Model file for the job. Use its own axes, mm. Face numbers are marked on the shaded views. A direction names the side the tool comes from. Give positions to 0.01 mm unless a question says otherwise; leave off trailing zeros. Loops run counter-clockwise (first coordinate to the right, second up) from the corner with the lowest first, then second, coordinate; pieces in that order, holes last. Notation, with made-up numbers: (-6.75, 56) - (1.25, 56) arc R28 ccw to (1.25, 75) - close; hole circle Ø1 at (58, 83.25). An arc over 180 degrees is marked (long way). Use a Markdown table: item, result.
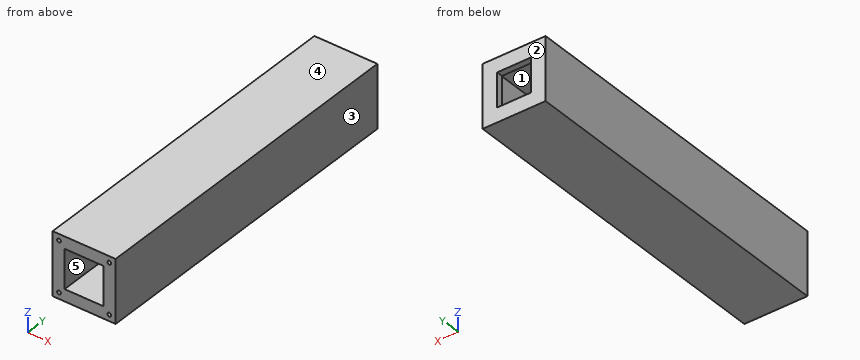
from build123d import *

# Parameters (mm, degrees)
SKETCH_1_W          = 10
SKETCH_1_H          = 10
SKETCH_1_W_2        = 6.2
SKETCH_1_H_2        = 6.2
EXTRUDE_1_DEPTH     = 54
EXTRUDE_START       = 54
SKETCH_1_3_W        = 10
SKETCH_1_3_H        = 10
SKETCH_1_3_W_2      = 6.2
SKETCH_1_3_H_2      = 6.2
SKETCH_1_3_W_3      = 5.4
SKETCH_1_3_H_3      = 5.4
EXTRUDE_2_DEPTH     = 1
SKETCH_2_R          = 0.3
CUT_EXTRUDE_1_DEPTH = 2


with BuildPart() as part:
    # 草图1 → 凸台-拉伸1 (new body)
    with BuildSketch(Plane(origin=(0, 0, 0), x_dir=(1, 0, 0), z_dir=(0, 1, 0))):
        Rectangle(SKETCH_1_W, SKETCH_1_H)
        Rectangle(SKETCH_1_W_2, SKETCH_1_H_2, mode=Mode.SUBTRACT)
    extrude(amount=EXTRUDE_1_DEPTH)

    # 草图1<3> → 凸台-拉伸2 (add)
    # profile 1 of 2: a face of its own
    with BuildSketch(Plane(origin=(0, 0, 0), x_dir=(1, 0, 0), z_dir=(0, 1, 0)).offset(EXTRUDE_START)):
        Rectangle(SKETCH_1_3_W, SKETCH_1_3_H)
        Rectangle(SKETCH_1_3_W_2, SKETCH_1_3_H_2, mode=Mode.SUBTRACT)
    # profile 2 of 2: a face of its own
    with BuildSketch(Plane(origin=(0, 0, 0), x_dir=(1, 0, 0), z_dir=(0, 1, 0)).offset(EXTRUDE_START)):
        Rectangle(SKETCH_1_3_W_2, SKETCH_1_3_H_2)
        Rectangle(SKETCH_1_3_W_3, SKETCH_1_3_H_3, mode=Mode.SUBTRACT)
    extrude(amount=-EXTRUDE_2_DEPTH)

    # 草图2 → 切除-拉伸1 (cut)
    with BuildSketch(Plane.XZ):
        with Locations(Location((-4, 4, 0), (0, 0, 270))):
            Circle(SKETCH_2_R)
        with Locations(Location((4, -4, 0), (0, 0, 270))):
            Circle(SKETCH_2_R)
        with Locations(Location((4, 4, 0), (0, 0, 270))):
            Circle(SKETCH_2_R)
        with Locations(Location((-4, -4, 0), (0, 0, 270))):
            Circle(SKETCH_2_R)
    extrude(amount=-CUT_EXTRUDE_1_DEPTH, mode=Mode.SUBTRACT)


solid = part.part
(1) Mould opens along X. For the marked faces 1, 2 and 3 say: pulls with the +X half, pulls with the -X half, needs draft (parallel to the pull), parting line crosses it, or undercut.
Computed:
| item | result |
|---|---|
| face 1 | undercut |
| face 2 | needs draft |
| face 3 | pulls with the +X half |
(2) Slice it at B-B, the plane z = 1.25. Write the cut outline in (x, y), plus the area to 3 significant figures.
Computed:
| item | result |
|---|---|
| outline | (-5, 0) - (-3.1, 0) - (-3.1, 53) - (-2.7, 53) - (-2.7, 54) - (-5, 54) - close; (2.7, 53) - (3.1, 53) - (3.1, 0) - (5, 0) - (5, 54) - (2.7, 54) - close |
| area | 206 mm² |
(3) Drill centre lines: probe 1 along X at (y, z) = (1.2, 4); probe 2 along X at (y, z) = (4.5, 0.5). Where is each one in solid material? Low to high. Write a range as [from, to].
Computed:
| item | result |
|---|---|
| probe 1 | [-5, -4.3], [-3.7, 3.7], [4.3, 5] |
| probe 2 | [-5, -3.1], [3.1, 5] |
(4) Slice it at C-C, the plane y = 5. Write the cut outline in (x, z), plus the area to 3 significant figures.
Computed:
| item | result |
|---|---|
| outline | (-5, -5) - (5, -5) - (5, 5) - (-5, 5) - close; hole (-3.1, -3.1) - (3.1, -3.1) - (3.1, 3.1) - (-3.1, 3.1) - close |
| area | 61.6 mm² |
(5) 3-axis set-ups, long thin cutter, end or side, ignore diameter. For the marked faces 4 and 5: which of +Z, -Z, +X, -X, +Y, -Y reach the whole face in a straight line?
Computed:
| item | result |
|---|---|
| face 4 | +Z, +X, -X, +Y, -Y |
| face 5 | -Y |
(6) Slice it at A-A, the plane x = -2.25. Write the cut outline in (y, z).
Computed:
| item | result |
|---|---|
| outline | (0, -5) - (54, -5) - (54, -2.7) - (53, -2.7) - (53, -3.1) - (0, -3.1) - close; (0, 3.1) - (53, 3.1) - (53, 2.7) - (54, 2.7) - (54, 5) - (0, 5) - close |
